from build123d import *

# Parameters (mm, degrees)
F0_R     = 20
F1_DEPTH = 30
F2_R     = 30
F3_DEPTH = 40
F4_R     = 60
F5_DEPTH = 180


with BuildPart() as f1:
    # F0 (on Top) → F1 (new body)
    with BuildSketch(Plane.XY):
        Circle(F0_R)
    extrude(amount=-F1_DEPTH)

    # F2 (on Top) → F3 (join)
    with BuildSketch(Plane.XY):
        Circle(F2_R)
    extrude(amount=F3_DEPTH)

    # F4 (on face) → F5 (join)
    with BuildSketch(Plane.XY.offset(40)):
        Circle(F4_R)
    extrude(amount=F5_DEPTH)


solid = f1.part
Input: part model. Units: mm. Frame: model coordinates. A direction names the side the tool comes from. Give positions to 0.01 mm unless a question says otherwise; leave off trailing zeros. Write each loop counter-clockwise with the first axis right and the second up, starting at its lowest first coordinate (ties: lowest second). Pieces come first, ordered by that corner, then holes.
Q1. Section A-A, the plane x = 0. Output: boundary loops of the cut face in (y, z).
Q2. Section D-D, the plane y = 24. Output: boundary loops of the cut face in (x, z).
Q3. Material intervals for probe 1 along Z at (x, y) = (24.5, -20); probe 2 along Z at (x, y) = (-24, 17.5); probe 3 along Y at (x, z) = (1, 164), sorted ascending.
Q4. Section C-C, the plane z = 44.5. Output: boundary loops of the cut face in (x, y), plus the area to 3 significant figures.
Q5. Set-up query: faces 1 (the face through (-59.94, 2.64, 128.74)), 2 (the face through (-4.336, -19.524, -14.79)). Return all of +Z, -Z, +X, -X, +Y, -Y with unobstructed straight access to the full face (end or side cutting, diameter ignored); none if empty.
Q6. First-contact query: P1, Ø8, axis at x = -22, z = 83.5, coming from the +Y side; P2, Ø5, axis at x = 4.5, z = 55, coming from the -Y side; P3, Ø5, axis at x = -35, z = 139, coming from the +Y side. Flat tips, straight axial feed; report the tip coordinate or a pass-through.
Filled in:
1. outline: (-60, 40) - (-30, 40) - (-30, 0) - (-20, 0) - (-20, -30) - (20, -30) - (20, 0) - (30, 0) - (30, 40) - (60, 40) - (60, 220) - (-60, 220) - close
2. outline: (-54.99, 40) - (-18, 40) - (-18, 0) - (18, 0) - (18, 40) - (54.99, 40) - (54.99, 220) - (-54.99, 220) - close
3. probe 1: z = 40 to 220
3. probe 2: z = 0 to 220
3. probe 3: y = -59.99 to 59.99
4. outline: circle Ø120 at (0, 0)
4. area: 11,300 mm2
5. face 1: +Z, -Z
5. face 2: -Z
6. P1: stops at y = 57.24
6. P2: stops at y = -59.97
6. P3: stops at y = 50.44
